from build123d import *

# Parameters (mm, degrees)
SKETCH_2_W          = 45
SKETCH_2_H          = 45
EXTRUDE_1_DEPTH     = 45
SKETCH_3_W          = 42
SKETCH_3_H          = 42
CUT_EXTRUDE_1_DEPTH = 30
CUT_EXTRUDE_2_REACH = 69.5
SKETCH_4_W          = 21
SKETCH_4_H          = 30
FILLET_2_R          = 3.5
FILLET_3_R          = 2


with BuildPart() as part:
    # 草图2 → 凸台-拉伸1 (new body)
    with BuildSketch(Plane.XY):
        Rectangle(SKETCH_2_W, SKETCH_2_H)
    extrude(amount=EXTRUDE_1_DEPTH)

    # 草图3 → 切除-拉伸1 (cut)
    with BuildSketch(Plane.XY.offset(45)):
        Rectangle(SKETCH_3_W, SKETCH_3_H)
    extrude(amount=-CUT_EXTRUDE_1_DEPTH, mode=Mode.SUBTRACT)

    # 草图4 → 切除-拉伸2 (cut, up to next)
    with BuildSketch(Plane.XZ.offset(22.5), mode=Mode.PRIVATE) as cut_extrude_2_sk1:
        with Locations((0, 30)):
            Rectangle(SKETCH_4_W, SKETCH_4_H)
    cut_extrude_2_tool1 = extrude(cut_extrude_2_sk1.sketch, amount=-CUT_EXTRUDE_2_REACH, mode=Mode.PRIVATE) & part.part
    add(cut_extrude_2_tool1.solids().sort_by_distance((0, -22.5, 30))[0], mode=Mode.SUBTRACT)

    # 圆角2
    fillet_2_edges = [part.edges().sort_by_distance(p)[0] for p in [
        (10.5, -21.75, 45),
        (-10.5, -21.75, 45),
    ]]
    fillet(fillet_2_edges, radius=FILLET_2_R)

    # 圆角3
    fillet_3_edges = [part.edges().sort_by_distance(p)[0] for p in [
        (0, -22.5, 0),
        (-22.5, 0, 0),
        (0, 22.5, 0),
        (22.5, 0, 0),
    ]]
    fillet(fillet_3_edges, radius=FILLET_3_R)


solid = part.part
Check sheet for the modelled part. Datum: model origin and axes. Units: mm. A direction names the side the tool comes from. Round coordinates to 2 decimals unless told otherwise and drop trailing zeros. Loops run counter-clockwise (first coordinate to the right, second up) from the corner with the lowest first, then second, coordinate; pieces in that order, holes last.
1. Gauge pin test, flat ends, axial feed: pin 1 Ø5 at (x, y) = (-7.5, 17.5) entering from +Z; pin 2 Ø24 at (x, z) = (0, 23) entering from -Y. Record the tip position at first contact, or that the pin passes through.
2. Sectioned sample at A-A on y = 17. Record the boundary of the cut face in (x, z), and give its area (3 significant figures).
3. Sectioned sample at C-C on z = 24. Record the boundary of the cut face in (x, y).
4. Set-up check for faces 4 (the flat face through (16, -21, 30)), 5 (the flat face through (-10.5, -22, 28)), 6 (the cylindrical face through (0.32, -21.93, 0.6)): record each of +Z, -Z, +X, -X, +Y, -Y from which the full face is reachable in a straight line by a thin tool's end or side.
5. Scan lines: probe 1 along X at (y, z) = (-9, 22); probe 2 along Z at (x, y) = (5.5, 1). Record each from-to range of solid material in increasing order.
6. Mould release check, pull along Y, two halves, no side actions. Record for faces 1 (the flat face through (-22.5, 0, 23)), 2 (the flat face through (0, 21, 30)), 3 (the flat face through (0, 22.5, 23)): released by +Y, released by -Y, zero draft, split by the parting line, or undercut.
7. Sectioned sample at B-B on x = 6.5. Record the boundary of the cut face in (y, z).
Recorded:
1. pin 1: stops at z = 15
1. pin 2: stops at y = -22.5
2. outline: (-22.5, 2) arc R2 ccw to (-20.5, 0) - (20.5, 0) arc R2 ccw to (22.5, 2) - (22.5, 45) - (21, 45) - (21, 15) - (-21, 15) - (-21, 45) - (-22.5, 45) - close
2. area: 763 mm2
3. outline: (-22.5, -22.5) - (-10.5, -22.5) - (-10.5, -21) - (-21, -21) - (-21, 21) - (21, 21) - (21, -21) - (10.5, -21) - (10.5, -22.5) - (22.5, -22.5) - (22.5, 22.5) - (-22.5, 22.5) - close
4. face 4: +Z
4. face 5: +Z, -Y
4. face 6: -Z, +X, -X, -Y
5. probe 1: x = -22.5 to -21, 21 to 22.5
5. probe 2: z = 0 to 15
6. face 1: zero draft
6. face 2: undercut
6. face 3: released by +Y
7. outline: (-22.5, 2) arc R2 ccw to (-20.5, 0) - (20.5, 0) arc R2 ccw to (22.5, 2) - (22.5, 45) - (21, 45) - (21, 15) - (-22.5, 15) - close
